```python
from build123d import *

# Parameters (mm, degrees)
F0_W     = 200
F0_H     = 4
F1_DEPTH = 175
F2_R     = 3.5
F3_DEPTH = 4


with BuildPart() as f1:
    # F0 (on Right) → F1 (new body, symmetric)
    with BuildSketch(Plane.YZ):
        with Locations((-100, 2)):
            Rectangle(F0_W, F0_H)
    extrude(amount=F1_DEPTH, both=True)

    # F2 (on face) → F3 (cut, through all)
    with BuildSketch(Plane.XY.offset(4)):
        with Locations((-145, -170)):
            Circle(F2_R)
        with Locations((-145, -30)):
            Circle(F2_R)
        with Locations((145, -30)):
            Circle(F2_R)
        with Locations((145, -170)):
            Circle(F2_R)
    extrude(amount=-F3_DEPTH, mode=Mode.SUBTRACT)


solid = f1.part
```
For this review, take the finished solid that the model builds, in its own axes (mm). Round coordinates to 2 decimals unless told otherwise and drop trailing zeros. Write each loop counter-clockwise with the first axis right and the second up, starting at its lowest first coordinate (ties: lowest second). Pieces come first, ordered by that corner, then holes. Notation, with made-up numbers: (-31, -6) - (6, -6) arc R17 cw to (6, 24) - close; hole circle Ø2 at (78, 62). An arc over 180 degrees is marked (long way). Write each question's results on one line, items separated by ' | '.
Item 1: Draft analysis for pull direction Y (two halves, no side actions). For faces 1 (the face through (-141.66, -28.95, 2.03)), 2 (the face through (-141.767, -171.341, 2.028)), 3 (the face through (2, -101, 0)), state which applies: pulls with the +Y half, pulls with the -Y half, needs draft (parallel to the pull), parting line crosses it, or undercut.
Calculated:
face 1: undercut | face 2: undercut | face 3: needs draft
Item 2: Take a section at A-A on x = 145. State the section outline as (y, z) points, then the cut area to 3 significant figures.
Calculated:
outline: (-200, 0) - (-173.5, 0) - (-173.5, 4) - (-200, 4) - close; (-166.5, 0) - (-33.5, 0) - (-33.5, 4) - (-166.5, 4) - close; (-26.5, 0) - (0, 0) - (0, 4) - (-26.5, 4) - close | area: 744 mm^2
Item 3: To check wall thickness, follow line 1 along Y through (x, z) = (145, 1.3); line 2 along X through (y, z) = (-170, 1.7); line 3 along Y through (x, z) = (-143, 2.25). State the ranges of each line that lie inside material, in increasing order. Write a range as from..to.
Calculated:
line 1: y = -200..-173.5, -166.5..-33.5, -26.5..0 | line 2: x = -175..-148.5, -141.5..141.5, 148.5..175 | line 3: y = -200..-172.87, -167.13..-32.87, -27.13..0
Item 4: Take a section at B-B on y = -170. State the section outline as (x, z) points, then the cut area to 3 significant figures.
Calculated:
outline: (-175, 0) - (-148.5, 0) - (-148.5, 4) - (-175, 4) - close; (-141.5, 0) - (141.5, 0) - (141.5, 4) - (-141.5, 4) - close; (148.5, 0) - (175, 0) - (175, 4) - (148.5, 4) - close | area: 1,340 mm^2
